Verification items for the finished model (mm, model axes). Face numbers are marked on the shaded views. Give positions to 0.01 mm unless a question says otherwise; leave off trailing zeros. Loops run counter-clockwise (first coordinate to the right, second up) from the corner with the lowest first, then second, coordinate; pieces in that order, holes last. Notation, with made-up numbers: M -39,-35.5 L -13,-35.5 A15 ccw -13,-29.5 Z; hole C 31,83.25 d4. An arc over 180 degrees is marked long. Answer in a Markdown table with one row per item.
Autodesk Inventor part; units mm, degrees
ref_plane "YZ Plane" through (0, 0, 0) normal (1, 0, 0) x (0, 1, 0)
ref_plane "XZ Plane" through (0, 0, 0) normal (0, 1, 0) x (-1, 0, 0)
ref_plane "XY Plane" through (0, 0, 0) normal (0, 0, 1) x (1, 0, 0)
sketch "Sketch1" plane through (0, 0, 0) normal (0, 1, 0) x (-1, 0, 0)
  circle A0 centre (0, 0) radius 6.45
  arc A1 (7.5, 0.8257) -> (-7.5, 0.8257) centre (0, 0.8257) ccw
  line L0 (-7.5, -5.5743) -> (-7.5, 0.8257)
  line L1 (7.5, -5.5743) -> (7.5, 0.8257)
  line L2 (7.5, -5.5743) -> (7.5, -9)
  line L3 (-7.5, -5.5743) -> (-7.5, -9)
  line L4 (7.5, -9) -> (-7.5, -9)
  dimension "d0" = 12.9
  dimension "d2" = 7.5
  dimension "d7" = 9
extrude "Extrusion1" add sketch "Sketch1" along normal blind 12
chamfer "Chamfer1" distance 2 angle 45 1 edges at (7.5, 6, -9)
chamfer "Chamfer2" distance 2 angle 45 1 edges at (-7.5, 6, -9)
properties part number "x bushing holder full"
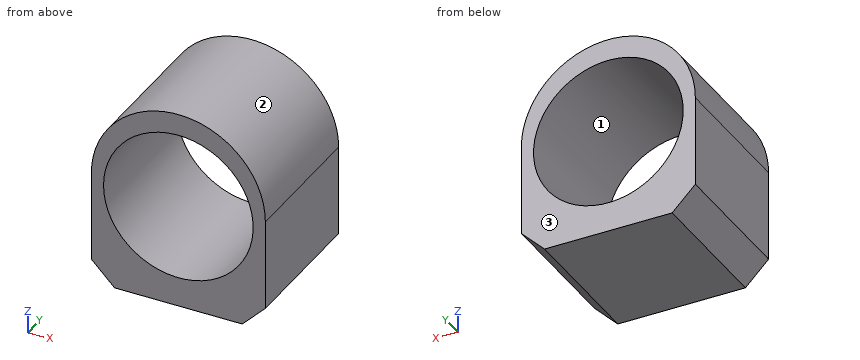
Item 1: Sectioned sample at C-C (y = 1.75). Record the cut outline in (x, z).
Reported:
| item | result |
|---|---|
| outline | M -7.5,-7 L -5.5,-9 L 5.5,-9 L 7.5,-7 L 7.5,0.83 A7.5 ccw -7.5,0.83 Z; hole C 0,0 d12.9 |
Item 2: Release check for a two-part mould opening along Z. For the marked faces 1, 2 and 3 record: released by +Z, released by -Z, zero draft, split by the parting line, or undercut.
Reported:
| item | result |
|---|---|
| face 1 | undercut |
| face 2 | released by +Z |
| face 3 | zero draft |
Item 3: Sectioned sample at B-B (z = 0). Record the cut outline in (x, y), and give its area (3 significant figures).
Reported:
| item | result |
|---|---|
| outline | M -7.5,0 L -6.45,0 L -6.45,12 L -7.5,12 Z; M 6.45,0 L 7.5,0 L 7.5,12 L 6.45,12 Z |
| area | 25.2 mm^2 |
Item 4: Sectioned sample at A-A (x = 0). Record the cut outline in (y, z), and give its area (3 significant figures).
Reported:
| item | result |
|---|---|
| outline | M 0,-9 L 12,-9 L 12,-6.45 L 0,-6.45 Z; M 0,6.45 L 12,6.45 L 12,8.33 L 0,8.33 Z |
| area | 53.1 mm^2 |
Item 5: Scan lines: L1, parallel to Z at x = 0, y = 5; L2, parallel to Z at x = -3, y = 10.75; L3, parallel to X at y = 5.5, z = 2.5. Record each from-to range of solid material in increasing order. Write a range as [from, to].
Reported:
| item | result |
|---|---|
| L1 | z = [-9, -6.45], [6.45, 8.33] |
| L2 | z = [-9, -5.71], [5.71, 7.7] |
| L3 | x = [-7.31, -5.95], [5.95, 7.31] |
Item 6: Sectioned sample at D-D (z = -7.25). Record the cut outline in (x, y).
Reported:
| item | result |
|---|---|
| outline | M -7.25,0 L 7.25,0 L 7.25,12 L -7.25,12 Z |
Item 7: Go/stop test with flat-tipped pins: pin 1 (6 mm diameter, centred on x = -0.5, y = 9.5, fed in from +Z); pin 2 (6 mm diameter, centred on x = -5, y = 8.5, fed in from +Z); pin 3 (2 mm diameter, centred on y = 1.5, z = 2, fed in from +X). Record where each tip stops, or that it passes through.
Reported:
| item | result |
|---|---|
| pin 1 | stops at z = 8.33 |
| pin 2 | stops at z = 8.05 |
| pin 3 | stops at x = 7.5 |
